Can you work these out from the drawing? Everything is in mm from the part's minimum corner. Round coordinates to 2 decimals unless told otherwise and drop trailing zeros. Loops run counter-clockwise (first coordinate to the right, second up) from the corner with the lowest first, then second, coordinate; pieces in that order, holes last. Notation, with made-up numbers: (25.25, 23.5) -> (64.25, 23.5) arc R25 ccw to (64.25, 38.5) -> close; hole circle Ø5 at (5.5, -31.75). An arc over 180 degrees is marked (long way). One line per item, written item: value.
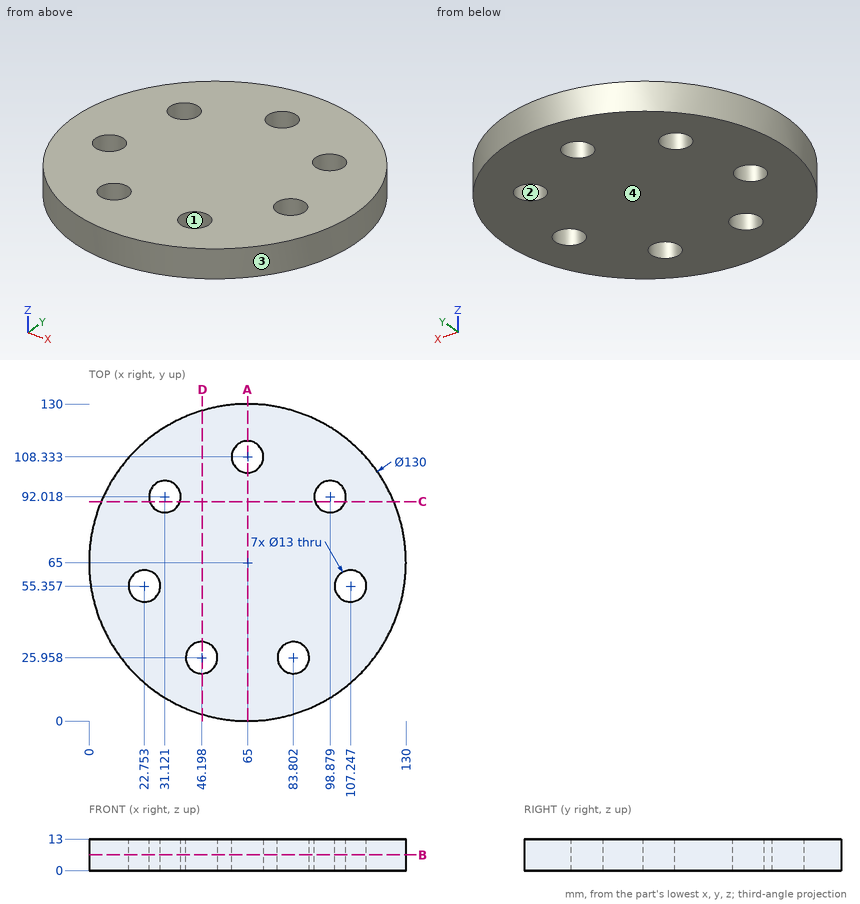
Item 1: If we section it at B-B on z = 6.5: List the corners of the cut face in (x, y) for me (1 decimal).
Output:
outline: circle Ø130 at (65, 65); hole circle Ø13 at (22.8, 55.4); hole circle Ø13 at (31.1, 92); hole circle Ø13 at (46.2, 26); hole circle Ø13 at (65, 108.3); hole circle Ø13 at (83.8, 26); hole circle Ø13 at (98.9, 92); hole circle Ø13 at (107.2, 55.4)
Item 2: If we section it at D-D on x = 46.5: List the corners of the cut face in (y, z) for me (1 decimal).
Output:
outline: (2.7, 0) -> (19.5, 0) -> (19.5, 13) -> (2.7, 13) -> close; (32.5, 0) -> (127.3, 0) -> (127.3, 13) -> (32.5, 13) -> close
Item 3: I need wall thicknesses on line 1 (X direction, y = 108, z = 7) (1 decimal); line 2 (X direction, y = 50, z = 5) (1 decimal); line 3 (Y direction, x = 65, z = 8). Which ranges of each line are inside material? Lowest first, please. Write a range as from..to.
Output:
line 1: x = 16.3..58.5, 71.5..113.7
line 2: x = 1.8..19.1, 26.4..103.6, 110.9..128.2
line 3: y = 0..101.83, 114.83..130
Item 4: If we section it at A-A on x = 65: List the corners of the cut face in (y, z) for me.
Output:
outline: (0, 0) -> (101.83, 0) -> (101.83, 13) -> (0, 13) -> close; (114.83, 0) -> (130, 0) -> (130, 13) -> (114.83, 13) -> close
Item 5: If we mould it in two halves opening along X, with no side actions, what happens to the marked faces 1, 2, 3 and 4? For each: released by +X, released by -X, zero draft, split by the parting line, or undercut.
Output:
face 1: undercut
face 2: undercut
face 3: split by the parting line
face 4: zero draft
Item 6: If we section it at C-C on y = 90: List the corners of the cut face in (x, z) for me.
Output:
outline: (5, 0) -> (24.94, 0) -> (24.94, 13) -> (5, 13) -> close; (37.3, 0) -> (92.7, 0) -> (92.7, 13) -> (37.3, 13) -> close; (105.06, 0) -> (125, 0) -> (125, 13) -> (105.06, 13) -> close
Item 7: Will these pins go through, and if not, where does the flat tip stop? pin 1 Ø5 at (x, z) = (112.5, 2) entering from +Y (1 decimal); pin 2 Ø3 at (x, z) = (104, 8.5) entering from -Y; pin 3 Ø1.5 at (x, z) = (101.5, 6.5) entering from +Y (1 decimal).
Output:
pin 1: stops at y = 111.9
pin 2: stops at y = 11.91
pin 3: stops at y = 119.3
